Here's how the part is built. I have some questions about the finished solid (model axes, mm). A direction names the side the tool comes from. Give positions to 0.01 mm unless a question says otherwise; leave off trailing zeros. Loops run counter-clockwise (first coordinate to the right, second up) from the corner with the lowest first, then second, coordinate; pieces in that order, holes last. Notation, with made-up numbers: (1, -34.5) - (13, -34.5) arc R19 ccw to (13, -7.5) - close; hole circle Ø4 at (0, 30.25). An arc over 180 degrees is marked (long way). Use a Markdown table: item, result.
from build123d import *

# Parameters (mm, degrees)
SKETCH1_W                  = 109
SKETCH1_H                  = 46
BOSS_EXTRUDE1_DEPTH        = 10
BOSS_EXTRUDE2_DEPTH        = 20
FILLET1_R                  = 5
CUT_EXTRUDE1_DEPTH         = 103.153071417
M5_TAPPED_HOLE2_AT_2_COUNT = 2
M5_TAPPED_HOLE2_AT_2_PITCH = 12
FILLET2_R                  = 2.5
FILLET3_R                  = 3


# Read off the part's stored shape, not the designer's step: M5 Tapped Hole1
with BuildPart() as part:
    # Sketch1 → Boss-Extrude1 (new body)
    with BuildSketch(Plane(origin=(0, 0, 0), x_dir=(1, 0, 0), z_dir=(0, 1, 0))):
        Rectangle(SKETCH1_W, SKETCH1_H)
    extrude(amount=-BOSS_EXTRUDE1_DEPTH)

    # Sketch1<3> → Boss-Extrude2 (add)
    with BuildSketch(Plane(origin=(0, 0, 0), x_dir=(1, 0, 0), z_dir=(0, 1, 0))):
        with BuildLine():
            Line((-54.5, -23), (-54.5, 23))
            Line((-54.5, 23), (-89.5, 23))
            Line((-89.5, 23), (-89.5, 14.7))
            Line((-89.5, 14.7), (-83.493997598, 14.7))
            ThreePointArc((-83.493997598, 14.7), (-61.930512441, -8.619716922), (-92.5, 0))
            Line((-92.5, 0), (-92.5, 23))
            Line((-92.5, 23), (-97.5, 23))
            Line((-97.5, 23), (-97.5, -15))
            ThreePointArc((-97.5, -15), (-95.156854249, -20.656854249), (-89.5, -23))
            Line((-89.5, -23), (-54.5, -23))
        make_face()
        with BuildLine():
            Line((92.5, 23), (92.5, 0))
            ThreePointArc((92.5, 0), (61.930512441, -8.619716922), (83.493997598, 14.7))
            Line((83.493997598, 14.7), (89.5, 14.7))
            Line((89.5, 14.7), (89.5, 23))
            Line((89.5, 23), (54.5, 23))
            Line((54.5, 23), (54.5, -23))
            Line((54.5, -23), (89.5, -23))
            ThreePointArc((89.5, -23), (95.156854249, -20.656854249), (97.5, -15))
            Line((97.5, -15), (97.5, 23))
            Line((97.5, 23), (92.5, 23))
        make_face()
    extrude(amount=-BOSS_EXTRUDE2_DEPTH)

    # Fillet1
    fillet1_edges = [part.edges().sort_by_distance(p)[0] for p in [
        (-54.5, -15, -23),
        (-54.5, -15, 23),
        (54.5, -15, 23),
        (54.5, -15, -23),
    ]]
    fillet(fillet1_edges, radius=FILLET1_R)

    # M5 Tapped Hole1 outline → M5 Tapped Hole1 (revolve, cut)
    with BuildSketch(Plane(origin=(48, 0, -15), x_dir=(1, 0, 0), z_dir=(0, 0, 1))):
        Polygon((0, -10), (2.1, -10), (2.1, -0.425), (2.525, 0), (0, 0), align=None)
    revolve(axis=Axis((48, 0, -15), (0, 1, 0)), mode=Mode.SUBTRACT)

    # M5 Tapped Hole1 2 outline → M5 Tapped Hole1 2 (revolve, cut)
    with BuildSketch(Plane(origin=(-48, 0, 15), x_dir=(1, 0, 0), z_dir=(0, 0, 1))):
        Polygon((0, -10), (2.1, -10), (2.1, -0.425), (2.525, 0), (0, 0), align=None)
    revolve(axis=Axis((-48, 0, 15), (0, 1, 0)), mode=Mode.SUBTRACT)

    # M5 Tapped Hole1 3 outline → M5 Tapped Hole1 3 (revolve, cut)
    with BuildSketch(Plane(origin=(-48, 0, -15), x_dir=(1, 0, 0), z_dir=(0, 0, 1))):
        Polygon((0, -10), (2.1, -10), (2.1, -0.425), (2.525, 0), (0, 0), align=None)
    revolve(axis=Axis((-48, 0, -15), (0, 1, 0)), mode=Mode.SUBTRACT)

    # M5 Tapped Hole1 4 outline → M5 Tapped Hole1 4 (revolve, cut)
    with BuildSketch(Plane(origin=(48, 0, 15), x_dir=(1, 0, 0), z_dir=(0, 0, 1))):
        Polygon((0, -10), (2.1, -10), (2.1, -0.425), (2.525, 0), (0, 0), align=None)
    revolve(axis=Axis((48, 0, 15), (0, 1, 0)), mode=Mode.SUBTRACT)

    # Sketch7 → Cut-Extrude1 (cut, through all)
    with BuildSketch(Plane(origin=(0, 0, 0), x_dir=(1, 0, 0), z_dir=(0, 1, 0))):
        Polygon((-31.298535282, 18), (31.298535282, 18), (0, 3), align=None)
        Polygon((-54.5, 4), (-54.5, -4), (-38.24, -18), (-0.681757662, 0), (-38.24, 18), align=None)
        Polygon((31.298535282, -18), (0, -3), (-31.298535282, -18), align=None)
        Polygon((38.24, -18), (0.681757662, 0), (38.24, 18), (54.5, 4), (54.5, -4), align=None)
    extrude(amount=-CUT_EXTRUDE1_DEPTH, mode=Mode.SUBTRACT)

    # Sketch9 → M5 Tapped Hole2 (revolve, cut)
    with BuildSketch(Plane(origin=(97.5, -4, -20), x_dir=(0, 0, -1), z_dir=(0, 1, 0))):
        Polygon((0, 0), (0, 17.2618073), (2.1, 16), (2.1, 0.425), (2.525, 0), align=None)
    m5_tapped_hole2 = revolve(axis=Axis((103.85, -4, -20), (-1, 0, 0)), mode=Mode.SUBTRACT)

    # M5 Tapped Hole2 at 2: M5 Tapped Hole2 ×2
    with Locations(*[(0, -i * M5_TAPPED_HOLE2_AT_2_PITCH, 0) for i in range(1, M5_TAPPED_HOLE2_AT_2_COUNT)]):
        add(m5_tapped_hole2, mode=Mode.SUBTRACT)

    # Mirror1: M5 Tapped Hole2 across plane
    add(m5_tapped_hole2.mirror(Plane(origin=(0, 0, 0), x_dir=(0, 0, 1), z_dir=(1, 0, 0))), mode=Mode.SUBTRACT)

    # Mirror1 copy 1 sketch → Mirror1 copy 1 (revolve, cut)
    with BuildSketch(Plane(origin=(-97.5, -16, -20), x_dir=(0, 0, -1), z_dir=(0, 1, 0))):
        Polygon((0, 0), (0, -17.2618073), (2.1, -16), (2.1, -0.425), (2.525, 0), align=None)
    revolve(axis=Axis((-103.85, -16, -20), (-1, 0, 0)), mode=Mode.SUBTRACT)

    # Fillet2
    fillet2_edges = [part.edges().sort_by_distance(p)[0] for p in [
        (31.298535282, -5, 18),
        (-31.298535282, -5, 18),
        (-0.681757662, -5, 0),
        (0.681757662, -5, 0),
        (-31.298535282, -5, -18),
        (31.298535282, -5, -18),
    ]]
    fillet(fillet2_edges, radius=FILLET2_R)

    # Fillet3
    fillet3_edges = [part.edges().sort_by_distance(p)[0] for p in [
        (0, -5, 3),
        (-38.24, -5, -18),
        (-54.5, -5, -4),
        (-38.24, -5, 18),
        (-54.5, -5, 4),
        (38.24, -5, 18),
        (54.5, -5, 4),
        (38.24, -5, -18),
        (54.5, -5, -4),
        (0, -5, -3),
    ]]
    fillet(fillet3_edges, radius=FILLET3_R)


solid = part.part
(1) If I drill on line 1 (Y direction, x = 93.6, z = -20); line 2 (X direction, y = -7.25, z = -9); line 3 (X direction, y = -5.5, z = -8.5), over which ranges is the centre line in solid material (lowest first)?
A:
| item | result |
|---|---|
| line 1 | -20 to -18.1, -13.9 to -6.1, -1.9 to 0 |
| line 2 | -97.5 to -92.5, -62.17 to -48.69, -19.46 to -12.52, 12.52 to 19.46, 48.69 to 62.17, 92.5 to 97.5 |
| line 3 | -97.5 to -92.5, -61.86 to -49.27, -18.42 to -11.48, 11.48 to 18.42, 49.27 to 61.86, 92.5 to 97.5 |
(2) Suppose I cut it at B-B on z = -7.5. Write out the boundary of the cut face in (x, y) (3 decimals).
A:
| item | result |
|---|---|
| outline | (-97.5, -20) - (-92.5, -20) - (-92.5, 0) - (-97.5, 0) - close; (-61.303, -20) - (-54.5, -20) - (-54.5, -10) - (-50.435, -10) - (-50.435, 0) - (-61.303, 0) - close; (-16.331, -10) - (-9.39, -10) - (-9.39, 0) - (-16.331, 0) - close; (9.39, -10) - (16.331, -10) - (16.331, 0) - (9.39, 0) - close; (50.435, -10) - (54.5, -10) - (54.5, -20) - (61.303, -20) - (61.303, 0) - (50.435, 0) - close; (92.5, -20) - (97.5, -20) - (97.5, 0) - (92.5, 0) - close |
(3) Suppose I cut it at C-C on x = -48. Write out the boundary of the cut face in (y, z) (3 decimals).
A:
| item | result |
|---|---|
| outline | (-10, -23) - (0, -23) - (0, -17.525) - (-0.425, -17.1) - (-10, -17.1) - close; (-10, -12.9) - (-0.425, -12.9) - (0, -12.475) - (0, -9.597) - (-10, -9.597) - close; (-10, 9.597) - (0, 9.597) - (0, 12.475) - (-0.425, 12.9) - (-10, 12.9) - close; (-10, 17.1) - (-0.425, 17.1) - (0, 17.525) - (0, 23) - (-10, 23) - close |
(4) Suppose I cut it at D-D on z = 10.5. Write out the boundary of the cut face in (x, y), plus the area to 3 significant figures.
A:
| item | result |
|---|---|
| outline | (-97.5, -20) - (-88.73, -20) - (-88.73, 0) - (-97.5, 0) - close; (-63.27, -20) - (-54.5, -20) - (-54.5, -10) - (-46.95, -10) - (-46.95, 0) - (-63.27, 0) - close; (-22.59, -10) - (-15.65, -10) - (-15.65, 0) - (-22.59, 0) - close; (15.65, -10) - (22.59, -10) - (22.59, 0) - (15.65, 0) - close; (46.95, -10) - (54.5, -10) - (54.5, -20) - (63.27, -20) - (63.27, 0) - (46.95, 0) - close; (88.73, -20) - (97.5, -20) - (97.5, 0) - (88.73, 0) - close |
| area | 992 mm2 |
(5) We'd pull the mould along Z, two halves only. Please class faces 1 (the face through (-1, 0, 0)), 2 (the face through (55.93, -15.07, -21.5)), 3 (the face through (86, -10, -14.7)): pulls with the +Z half, pulls with the -Z half, needs draft (parallel to the pull), parting line crosses it, or undercut.
A:
| item | result |
|---|---|
| face 1 | needs draft |
| face 2 | pulls with the -Z half |
| face 3 | undercut |
(6) Suppose I cut it at A-A on x = -76. Write out the boundary of the cut face in (y, z), plus the area to 3 significant figures.
A:
| item | result |
|---|---|
| outline | (-20, -23) - (0, -23) - (0, -16.5) - (-20, -16.5) - close; (-20, 16.5) - (0, 16.5) - (0, 23) - (-20, 23) - close |
| area | 260 mm2 |
(7) Will these pins go through, and if not, where does the flat tip stop? pin 1 (3.5 mm diameter, centred on y = -4, z = -20, fed in from +X); pin 2 (2 mm diameter, centred on x = -40, z = -17.5, fed in from -Y); pin 3 (5 mm diameter, centred on y = -16, z = -20, fed in from +X) (3 decimals).
A:
| item | result |
|---|---|
| pin 1 | x = 81.29 |
| pin 2 | y = -10 |
| pin 3 | x = 97.475 |
(8) On a 3-axis mill with a long thin cutter (end or side, diameter ignored), from which of +Z, -Z, +X, -X, +Y, -Y can I reach the whole of each face in a straight line? I mean faces 4 (the face through (85.556, -18.082, -19.727)), 5 (the face through (0, -5, -18)), 6 (the face through (-55.93, -15.07, -21.5)), 7 (the face through (-89.5, -10, -19)). Say none if no direction works.
A:
| item | result |
|---|---|
| face 4 | +X |
| face 5 | +Y, -Y |
| face 6 | -Z, -Y |
| face 7 | -Z, +Y, -Y |
